Geometry: final body of the model. Coordinates: model frame, mm. A direction names the side the tool comes from. Coordinates: 2 decimals unless noted, no trailing zeros. Order: outer loops, then holes, each group sorted by start corner. A loop starts at its lowest first (then second) coordinate and runs counter-clockwise, first axis right, second up. Notation, with made-up numbers: (14, -27.75) -> (31, -27.75) arc R23 ccw to (31, -17.75) -> close; hole circle Ø2 at (72, 45). An arc over 180 degrees is marked (long way). Answer in a Markdown table with one row per item. Add a question column.
1) Ray query, line 1 (Z direction, x = 36.5, y = 66.5) (3 decimals); line 2 (X direction, y = -1.5, z = 2.5) (3 decimals); line 3 (X direction, y = 4, z = 3) (3 decimals). Return the intervals inside material, ascending. Write a range as from..to.
2) Pull-direction query (X, two-part tool) for faces 5 (the face through (60, -27, 9.525)), 6 (the face through (14, 12, 3.175)), 7 (the face through (3.46, 82.477, 0.133)); classes: +X half, -X half, draft (parallel to the pull), parting line (faces both ways), or undercut.
3) Set-up query: faces 1 (the face through (66.06, -10.39, 6.39)), 2 (the face through (12.065, -33, -2)), 3 (the face through (39.37, 67, 6)), 4 (the face through (-63, -21, 9.525)). Return all of +Z, -Z, +X, -X, +Y, -Y with unobstructed straight access to the full face (end or side cutting, diameter ignored); none if empty.
4) Contact query for flat-ended pins moving along their axis: P1, Ø1, axis at x = 55, y = -10.5, coming from the +Z side (3 decimals); P2, Ø1, axis at y = 56.5, z = 2.5, coming from the -X side; P3, Ø4, axis at x = 7, z = 1, coming from the -Y side. Output: stop coordinate, or through.
5) Section query B-B on y = 0. Return the cut outline in (x, z) (3 decimals), then the cut area to 3 significant figures.
6) Section query A-A on z = 5.5. Return the cut outline in (x, y) (3 decimals).
7) Section query D-D on x = 56.5. Return the cut outline in (y, z) (3 decimals), then the cut area to 3 significant figures.
8) Section query C-C on y = -30. Return the cut outline in (x, z) (3 decimals).
```python
from build123d import *

# Parameters (mm, degrees)
F0_R     = 82.55
F1_DEPTH = 9.525
F2_W     = 24.13
F2_H     = 99.441
F3_DEPTH = 9.525
F5_R     = 67.945
F6_DEPTH = 6.35
F8_DEPTH = 6.35


with BuildPart() as f1:
    # F0 (on Top) → F1 (new body, symmetric)
    with BuildSketch(Plane.XY):
        Circle(F0_R)
    extrude(amount=F1_DEPTH, both=True)

    # F2 (on Top) → F3 (cut, symmetric)
    with BuildSketch(Plane.XY):
        with Locations((0, -32.900974)):
            Rectangle(F2_W, F2_H)
    extrude(amount=F3_DEPTH, both=True, mode=Mode.SUBTRACT)

    # F5 (on face) → F6 (cut)
    with BuildSketch(Plane.XY.offset(9.525)):
        with Locations((0, 5.5118)):
            Circle(F5_R)
    extrude(amount=-F6_DEPTH, mode=Mode.SUBTRACT)

    # F7 (on offset) → F8 (cut)
    with BuildSketch(Plane(origin=(0, 4.112923, 9.525), x_dir=(1, 0, 0), z_dir=(0, 0, 1))):
        Polygon((39.37, 103.543088), (6.096, 103.543088), (-38.608, 103.543088), (-38.608, 52.743088), (39.37, 52.743088), align=None)
    extrude(amount=-F8_DEPTH, mode=Mode.SUBTRACT)


solid = f1.part
```
Result:
| question | item | result |
|---|---|---|
| 1 | line 1 | -9.525..3.175 |
| 1 | line 2 | -82.536..-12.065, 12.065..82.536 |
| 1 | line 3 | -82.453..-12.065, 12.065..82.453 |
| 2 | face 5 | draft |
| 2 | face 6 | undercut |
| 2 | face 7 | parting line |
| 3 | face 1 | +Z |
| 3 | face 2 | +Z, -Z, -Y |
| 3 | face 3 | +Z, +Y |
| 3 | face 4 | +Z, +X, -X, +Y, -Y |
| 4 | P1 | z = 3.175 |
| 4 | P2 | x = -60.65 |
| 4 | P3 | y = 16.82 |
| 5 | outline | (-82.55, -9.525) -> (-12.065, -9.525) -> (-12.065, 3.175) -> (-67.721, 3.175) -> (-67.721, 9.525) -> (-82.55, 9.525) -> close; (12.065, -9.525) -> (82.55, -9.525) -> (82.55, 9.525) -> (67.721, 9.525) -> (67.721, 3.175) -> (12.065, 3.175) -> close |
| 5 | area | 1,980 mm2 |
| 6 | outline | (-38.608, 61.422) -> (-38.608, 72.965) arc R82.55 ccw to (-12.065, -81.664) -> (-12.065, -61.353) arc R67.945 cw to start; (12.065, -81.664) arc R82.55 ccw to (39.37, 72.557) -> (39.37, 60.888) arc R67.945 cw to (12.065, -61.353) -> close |
| 7 | outline | (-60.185, -9.525) -> (60.185, -9.525) -> (60.185, 9.525) -> (43.251, 9.525) -> (43.251, 3.175) -> (-32.228, 3.175) -> (-32.228, 9.525) -> (-60.185, 9.525) -> close |
| 7 | area | 1,810 mm2 |
| 8 | outline | (-76.906, -9.525) -> (-12.065, -9.525) -> (-12.065, 3.175) -> (-57.926, 3.175) -> (-57.926, 9.525) -> (-76.906, 9.525) -> close; (12.065, -9.525) -> (76.906, -9.525) -> (76.906, 9.525) -> (57.926, 9.525) -> (57.926, 3.175) -> (12.065, 3.175) -> close |
